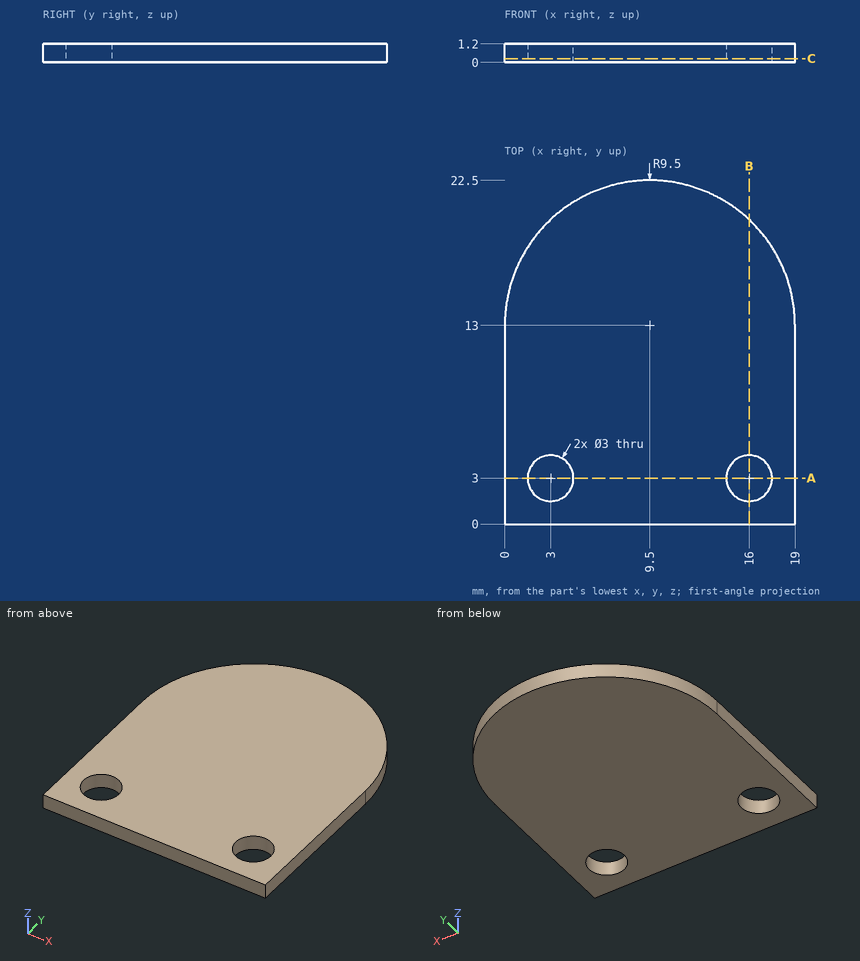
Job drawing, mm, ordinate dimensions from the low corner. One solid piece. Round coordinates to 2 decimals unless told otherwise and drop trailing zeros. Write each loop counter-clockwise with the first axis right and the second up, starting at its lowest first coordinate (ties: lowest second). Pieces come first, ordered by that corner, then holes.
1) Drill centre lines: probe 1 along X at (y, z) = (3.5, 0.65); probe 2 along Y at (x, z) = (16.25, 0.4); probe 3 along Y at (x, z) = (3, 0.8). Where is each one in solid material? Low to high.
2) Pin check, flat tips, straight feed: pin 1 (2.5 mm diameter, centred on x = 16, y = 3, fed in from -Z); pin 2 (4 mm diameter, centred on x = 8.5, y = 5, fed in from -Z). Stop position of each tip, or through.
3) Band-saw the part on A-A, the plane y = 3. List the corners of the cut face in (x, z).
4) Band-saw the part on B-B, the plane x = 16. List the corners of the cut face in (y, z), and give its area (3 significant figures).
5) Band-saw the part on C-C, the plane z = 0.25. List the corners of the cut face in (x, y).
Ans:
1. probe 1: x = 0 to 1.59, 4.41 to 14.59, 17.41 to 19
1. probe 2: y = 0 to 1.52, 4.48 to 19.68
1. probe 3: y = 0 to 1.5, 4.5 to 19.93
2. pin 1: passes through
2. pin 2: stops at z = 0
3. outline: (0, 0) - (1.5, 0) - (1.5, 1.2) - (0, 1.2) - close; (4.5, 0) - (14.5, 0) - (14.5, 1.2) - (4.5, 1.2) - close; (17.5, 0) - (19, 0) - (19, 1.2) - (17.5, 1.2) - close
4. outline: (0, 0) - (1.5, 0) - (1.5, 1.2) - (0, 1.2) - close; (4.5, 0) - (19.93, 0) - (19.93, 1.2) - (4.5, 1.2) - close
4. area: 20.3 mm2
5. outline: (0, 0) - (19, 0) - (19, 13) arc R9.5 ccw to (0, 13) - close; hole circle Ø3 at (3, 3); hole circle Ø3 at (16, 3)
